from build123d import *

# Parameters (mm, degrees)
F1_DEPTH = 11.1375302076
F3_DEPTH = 25.4


# Not quite as in the source:
# - a feature names something its author has since deleted; it is built from what else it names


with BuildPart() as f1:
    # F0 (on Front) → F1 (new body, symmetric)
    with BuildSketch(Plane.XZ):
        Polygon((-47.7266, 0), (0, 0), (0, 33.5543528199), (-66.2321434704, 33.5543528199), (-66.2321434704, 0), align=None)
        Polygon((47.7266, 0), (0, 0), (0, -26.3268053532), (23.8633, -26.3268053532), (47.7266, -26.3268053532), align=None)
        Polygon((0, 33.5543528199), (0, 0), (47.7266, 0), (66.2432, 0), (66.2432, 33.5543528199), align=None)
        Polygon((0, -26.3268053532), (0, 0), (-47.7266, 0), (-47.7266, -26.3268053532), (-23.8633, -26.3268053532), align=None)
    extrude(amount=F1_DEPTH, both=True)

    # F2 (on face) → F3 (join)
    with BuildSketch(Plane.XZ.offset(11.1375302076)):
        Polygon((-21.9350446656, 23.558561476), (-26.957899332, 27.1239373833), (-37.0000749826, 2.6461503003), (-30.5145010352, 2.6461503003), (-26.2247728504, 13.1023558882), align=None)
        Polygon((-21.9350446656, 27.1239373833), (-26.957899332, 27.1239373833), (-21.9350446656, 23.558561476), (-17.1249434352, 13.1023558882), (-13.4637281299, 2.6461503003), (-9.2794969678, 2.6461503003), align=None)
        Polygon((-17.1249434352, 13.1023558882), (-21.9350446656, 23.558561476), (-26.2247728504, 13.1023558882), align=None)
        with BuildLine():
            ThreePointArc((21.8997799497, 15.7127540144), (21.0422650014, 12.6276476595), (18.7955158738, 10.3461281077))
            Line((18.7955158738, 10.3461281077), (23.2909736673, 2.8426809347))
            ThreePointArc((23.2909736673, 2.8426809347), (25.5526183138, 4.5004893654), (27.4696294265, 6.5470556834))
            Line((27.4696294265, 6.5470556834), (21.9791319159, 15.7113410392))
            Line((21.9791319159, 15.7113410392), (21.8997799497, 15.7127540144))
        make_face()
        with BuildLine():
            Line((23.2909736673, 2.8426809347), (18.7955158738, 10.3461281077))
            ThreePointArc((18.7955158738, 10.3461281077), (9.9537248959, 18.9759861326), (21.9007925331, 15.8264953643))
            ThreePointArc((21.9007925331, 15.8264953643), (21.9005393822, 15.7696224358), (21.8997799497, 15.7127540144))
            Line((21.8997799497, 15.7127540144), (21.9791319159, 15.7113410392))
            Line((21.9791319159, 15.7113410392), (27.4696294265, 6.5470556834))
            ThreePointArc((27.4696294265, 6.5470556834), (29.8312607656, 10.9221852492), (30.6478411926, 15.8264953643))
            ThreePointArc((30.6478411926, 15.8264953643), (2.3434407909, 23.2881127649), (23.2909736673, 2.8426809347))
        make_face()
        with BuildLine():
            ThreePointArc((27.4696294265, 6.5470556834), (25.5526183138, 4.5004893654), (23.2909736673, 2.8426809347))
            Line((23.2909736673, 2.8426809347), (29.7385305166, -7.9190488905))
            Line((29.7385305166, -7.9190488905), (34.4466119702, -5.0983478214))
            Line((34.4466119702, -5.0983478214), (27.4696294265, 6.5470556834))
        make_face()
        with BuildLine():
            Line((21.8997799497, 15.7127540144), (15.512123704, 15.8264953643))
            Line((15.512123704, 15.8264953643), (18.7955158738, 10.3461281077))
            ThreePointArc((18.7955158738, 10.3461281077), (21.0422650014, 12.6276476595), (21.8997799497, 15.7127540144))
        make_face()
    extrude(amount=F3_DEPTH)


solid = f1.part
Here's how the part is built. I have some questions about the finished solid (model axes, mm). A direction names the side the tool comes from. Coordinates: 2 decimals unless noted, no trailing zeros. Order: outer loops, then holes, each group sorted by start corner. A loop starts at its lowest first (then second) coordinate and runs counter-clockwise, first axis right, second up.
Item 1: If we section it at D-D on x = -41: List the corners of the cut face in (y, z) for me, plus the area to 3 significant figures.
Result sheet:
outline: (-11.14, -26.33) - (11.14, -26.33) - (11.14, 33.55) - (-11.14, 33.55) - close
area: 1,330 mm2
Item 2: I need wall thicknesses on line 1 (X direction, y = -24, z = 20); line 2 (X direction, y = -29.5, z = 16); line 3 (X direction, y = -4, z = -7). Which ranges of each line are inside material? Lowest first, please.
Result sheet:
line 1: x = -29.88 to -18.25, 0.96 to 10.68, 20.35 to 30.06
line 2: x = -31.52 to -16.18, 0.38 to 9.13, 21.9 to 30.65
line 3: x = -47.73 to 47.73
Item 3: For P1, Ø10, axis at x = 22, y = -27.5, coming from the -Z side; P2, Ø5, axis at x = 27, y = -15.5, coming from the +Z side; P3, Ø10, axis at x = -22, y = -23.5, coming from the -Z side, each with a flat end and sliding along its axis, tell me the tip position at first contact or that it passes through.
Result sheet:
P1: stops at z = -3.35
P2: stops at z = 28
P3: stops at z = 11.21
Item 4: If we mould it in two halves opening along Z, with no side actions, what happens to faces 1 (the face through (-1, 11.138, 4)), 2 (the face through (-15.519, -23.66, 14.714)), 3 (the face through (57, 0, 0)), 4 (the face through (31.01, -23.66, 0.64))? For each: +Z half, -Z half, draft (parallel to the pull), parting line (faces both ways), or undercut.
Result sheet:
face 1: draft
face 2: +Z half
face 3: -Z half
face 4: undercut
Item 5: If we section it at A-A on y = -22: List the corners of the cut face in (x, z) for me.
Result sheet:
outline: (-37, 2.65) - (-30.51, 2.65) - (-26.22, 13.1) - (-17.12, 13.1) - (-13.46, 2.65) - (-9.28, 2.65) - (-21.94, 27.12) - (-26.96, 27.12) - close; (23.29, 2.84) - (29.74, -7.92) - (34.45, -5.1) - (27.47, 6.55) arc R15.14 ccw (long way) to start; hole (15.51, 15.83) - (21.9, 15.71) arc R6.39 ccw (long way) to (18.8, 10.35) - close
Item 6: If we section it at C-C on z = 19.5: List the corners of the cut face in (x, y) for me.
Result sheet:
outline: (-66.23, -11.14) - (-30.09, -11.14) - (-30.09, -36.54) - (-17.99, -36.54) - (-17.99, -11.14) - (0.83, -11.14) - (0.83, -36.54) - (10.29, -36.54) - (10.29, -11.14) - (20.74, -11.14) - (20.74, -36.54) - (30.2, -36.54) - (30.2, -11.14) - (66.24, -11.14) - (66.24, 11.14) - (-66.23, 11.14) - close
Item 7: If we section it at B-B on y = -0.5: List the corners of the cut face in (x, z) for me, plus the area to 3 significant figures.
Result sheet:
outline: (-66.23, 0) - (-47.73, 0) - (-47.73, -26.33) - (47.73, -26.33) - (47.73, 0) - (66.24, 0) - (66.24, 33.55) - (-66.23, 33.55) - close
area: 6,960 mm2
Item 8: For faces 5 (the face through (-11, -24, 2.646)), 6 (the face through (32.06, -23.66, -6.53)), 7 (the face through (-31.909, -23.66, 15.056)), 8 (the face through (-57, 0, 0)), 9 (the face through (-22, -24, 13.102)), which set-ups out of +Z, -Z, +X, -X, +Y, -Y let a thin tool reach every point of the face, with its end or its side?
Result sheet:
face 5: -Z, -X, -Y
face 6: -Z, +X, -Y
face 7: +Z, -X, -Y
face 8: -Z, -X, +Y, -Y
face 9: -Z, -Y
